```python
from build123d import *

# Parameters (mm, degrees)
SKETCH1_W               = 390
SKETCH1_H               = 120
SKETCH1_R               = 3.2
BOSS_EXTRUDE1_DEPTH     = 2.03
EDGE_FLANGE1_DEPTH      = 120
EDGE_FLANGE1_BEND_DEPTH = 120
CUT_EXTRUDE1_REACH      = 210.681
CUT_EXTRUDE2_DEPTH      = 209.447861347
CUT_EXTRUDE2_DEPTH_BACK = 209.447861347
SKETCH19_R              = 2.5
SKETCH20_R              = 3.35
CUT_EXTRUDE3_DEPTH      = 209.447861347
SKETCH21_R              = 3.175
CUT_EXTRUDE4_DEPTH      = 209.681312053


# Sheet-metal steps are written as plain solids
with BuildPart() as part:
    # Sketch1 → Boss-Extrude1 (new body)
    with BuildSketch(Plane(origin=(0, 0, 0), x_dir=(1, 0, 0), z_dir=(0, 1, 0))):
        Rectangle(SKETCH1_W, SKETCH1_H)
        with Locations(Location((0, 50, 0), (0, 0, 270))):
            Circle(SKETCH1_R, mode=Mode.SUBTRACT)
        with Locations(Location((-185, 50, 0), (0, 0, 270))):
            Circle(SKETCH1_R, mode=Mode.SUBTRACT)
        with Locations(Location((-185, -50, 0), (0, 0, 270))):
            Circle(SKETCH1_R, mode=Mode.SUBTRACT)
        with Locations(Location((0, -50, 0), (0, 0, 270))):
            Circle(SKETCH1_R, mode=Mode.SUBTRACT)
        with Locations(Location((185, -50, 0), (0, 0, 270))):
            Circle(SKETCH1_R, mode=Mode.SUBTRACT)
        with Locations(Location((185, 50, 0), (0, 0, 270))):
            Circle(SKETCH1_R, mode=Mode.SUBTRACT)
    extrude(amount=-BOSS_EXTRUDE1_DEPTH)

    # Edge-Flange1 section (across the edge) → Edge-Flange1 (add)
    with BuildSketch(Plane(origin=(-196.27, 0, -60), x_dir=(1, 0, 0), z_dir=(0, 0, 1))):
        with BuildLine():
            Line((-2.03, 1.27), (-2.03, 22.97))
            Line((-2.03, 22.97), (0, 22.97))
            Line((0, 22.97), (0, 1.27))
            ThreePointArc((0, 1.27), (0.371974388, 0.371974388), (1.27, 0))
            Line((1.27, 0), (1.27, -2.03))
            ThreePointArc((1.27, -2.03), (-1.063452378, -1.063452378), (-2.03, 1.27))
        make_face()
    extrude(amount=EDGE_FLANGE1_DEPTH)

    # Edge-Flange1 section 2 (across the edge) → Edge-Flange1 bend (add)
    with BuildSketch(Plane(origin=(196.27, 0, 60), x_dir=(-1, 0, 0), z_dir=(0, 0, -1))):
        with BuildLine():
            Line((-2.03, 1.27), (-2.03, 22.97))
            Line((-2.03, 22.97), (0, 22.97))
            Line((0, 22.97), (0, 1.27))
            ThreePointArc((0, 1.27), (0.371974388, 0.371974388), (1.27, 0))
            Line((1.27, 0), (1.27, -2.03))
            ThreePointArc((1.27, -2.03), (-1.063452378, -1.063452378), (-2.03, 1.27))
        make_face()
    extrude(amount=EDGE_FLANGE1_BEND_DEPTH)

    # Sketch18 → Cut-Extrude1 (cut, up to next)
    with BuildSketch(Plane.XZ.offset(2.03), mode=Mode.PRIVATE) as cut_extrude1_sk1:
        with BuildLine():
            Line((-157.5, -37.5), (-27.5, -37.5))
            ThreePointArc((-27.5, -37.5), (-23.964466094, -36.035533906), (-22.5, -32.5))
            Line((-22.5, -32.5), (-22.5, 32.5))
            ThreePointArc((-22.5, 32.5), (-23.964466094, 36.035533906), (-27.5, 37.5))
            Line((-27.5, 37.5), (-157.5, 37.5))
            ThreePointArc((-157.5, 37.5), (-161.035533906, 36.035533906), (-162.5, 32.5))
            Line((-162.5, 32.5), (-162.5, -32.5))
            ThreePointArc((-162.5, -32.5), (-161.035533906, -36.035533906), (-157.5, -37.5))
        make_face()
    cut_extrude1_tool1 = extrude(cut_extrude1_sk1.sketch, amount=-CUT_EXTRUDE1_REACH, mode=Mode.PRIVATE) & part.part
    # Sketch18 → Cut-Extrude1 (cut, up to next)
    with BuildSketch(Plane.XZ.offset(2.03), mode=Mode.PRIVATE) as cut_extrude1_sk2:
        with BuildLine():
            Line((22.5, -32.5), (22.5, 32.5))
            ThreePointArc((22.5, 32.5), (23.964466094, 36.035533906), (27.5, 37.5))
            Line((27.5, 37.5), (157.5, 37.5))
            ThreePointArc((157.5, 37.5), (161.035533906, 36.035533906), (162.5, 32.5))
            Line((162.5, 32.5), (162.5, -32.5))
            ThreePointArc((162.5, -32.5), (161.035533906, -36.035533906), (157.5, -37.5))
            Line((157.5, -37.5), (27.5, -37.5))
            ThreePointArc((27.5, -37.5), (23.964466094, -36.035533906), (22.5, -32.5))
        make_face()
    cut_extrude1_tool2 = extrude(cut_extrude1_sk2.sketch, amount=-CUT_EXTRUDE1_REACH, mode=Mode.PRIVATE) & part.part
    add(cut_extrude1_tool1.solids().sort_by_distance((-92.5, -2.03, 0))[0], mode=Mode.SUBTRACT)
    add(cut_extrude1_tool2.solids().sort_by_distance((92.5, -2.03, 0))[0], mode=Mode.SUBTRACT)

    # Sketch19 → Cut-Extrude2 (cut, two sides: drawn at the far end of the back side and taken through both)
    with BuildSketch(Plane(origin=(0, 0, 0), x_dir=(0, 0, -1), z_dir=(1, 0, 0)).offset(-CUT_EXTRUDE2_DEPTH_BACK)):
        with Locations((-47.5, 15.65)):
            Circle(SKETCH19_R)
        with Locations((0, 15.65)):
            Circle(SKETCH19_R)
        with Locations((47.5, 15.65)):
            Circle(SKETCH19_R)
    extrude(amount=CUT_EXTRUDE2_DEPTH + CUT_EXTRUDE2_DEPTH_BACK, mode=Mode.SUBTRACT)

    # Sketch20 → Cut-Extrude3 (cut, through all)
    with BuildSketch(Plane(origin=(0, 0, 0), x_dir=(1, 0, 0), z_dir=(0, 1, 0))):
        with Locations(Location((-92.5, -48.75, 0), (0, 0, 270))):
            Circle(SKETCH20_R)
        with Locations(Location((92.5, -48.75, 0), (0, 0, 90))):
            Circle(SKETCH20_R)
        with Locations(Location((92.5, 48.75, 0), (0, 0, 270))):
            Circle(SKETCH20_R)
        with Locations(Location((-92.5, 48.75, 0), (0, 0, 90))):
            Circle(SKETCH20_R)
    extrude(amount=-CUT_EXTRUDE3_DEPTH, mode=Mode.SUBTRACT)

    # Sketch21 → Cut-Extrude4 (cut, through all)
    with BuildSketch(Plane.XZ.offset(2.03)):
        with Locations(Location((-180, 0, 0), (0, 0, 270))):
            Circle(SKETCH21_R)
    extrude(amount=-CUT_EXTRUDE4_DEPTH, mode=Mode.SUBTRACT)


solid = part.part
```
Work out the finished part from the listing and answer in its coordinate system (mm). A direction names the side the tool comes from. Give positions to 0.01 mm unless a question says otherwise; leave off trailing zeros. Order: outer loops, then holes, each group sorted by start corner. A loop starts at its lowest first (then second) coordinate and runs counter-clockwise, first axis right, second up. Notation, with made-up numbers: (-29.5, 77) - (-24.5, 77) arc R25 cw to (-24.5, 114) - close; hole circle Ø2 at (-6.75, -16). An arc over 180 degrees is marked (long way). One line per item, written item: value. Start each with the question number.
1. Section B-B, the plane x = 92.5 is taken. Write down the section's boundary in (y, z), then the cut area to 3 significant figures.
2. Each of these flat-tipped pins is pushed along its axis until it touches: pin 1 Ø10 at (x, z) = (-180, 0) entering from +Y; pin 2 Ø0.6 at (y, z) = (-0.5, -11) entering from +X; pin 3 Ø1.6 at (y, z) = (-1, -3) entering from -X. Where does it stop, or does it pass through?
3. Section A-A, the plane x = -153 is taken. Write down the section's boundary in (y, z).
4. Consider line 1 (Z direction, x = -197.2, y = 15.65); line 2 (X direction, y = 1.5, z = -9); line 3 (Z direction, x = 185, y = -0.65). Determine where each line is inside the solid, lowest interval first.
5. Which of the six approach directions +Z, -Z, +X, -X, +Y, -Y give full straight-line access (tool end or side, diameter ignored) to faces 5 (the face through (196.27, 12, 1)), 6 (the face through (-3, -2.03, -1))?
6. Section C-C, the plane y = 6.75 is taken. Write down the section's boundary in (x, z).
7. For a pull along Z with two mould halves and no side action, classify faces 1 (the face through (188.173, -1.001, 49.583)), 2 (the face through (-1, -1, 60)), 3 (the face through (-176.85, -1.03, 0.41)), 4 (the face through (-3, 0, -1)) as released by +Z, released by -Z, zero draft, split by the parting line, or undercut.
Filled sheet:
1. outline: (-2.03, -60) - (0, -60) - (0, -52.1) - (-2.03, -52.1) - close; (-2.03, -45.4) - (0, -45.4) - (0, -37.5) - (-2.03, -37.5) - close; (-2.03, 37.5) - (0, 37.5) - (0, 45.4) - (-2.03, 45.4) - close; (-2.03, 52.1) - (0, 52.1) - (0, 60) - (-2.03, 60) - close
1. area: 64.1 mm²
2. pin 1: y = 0
2. pin 2: x = 197.95
2. pin 3: x = -197.95
3. outline: (-2.03, -60) - (0, -60) - (0, -37.5) - (-2.03, -37.5) - close; (-2.03, 37.5) - (0, 37.5) - (0, 60) - (-2.03, 60) - close
4. line 1: -60 to -50, -45 to -2.5, 2.5 to 45, 50 to 60
4. line 2: -198.3 to -196.27, 196.27 to 198.3
4. line 3: -60 to -53.2, -46.8 to 46.8, 53.2 to 60
5. face 5: +Z, -Z, +Y
5. face 6: +Z, -Z, +X, -X, -Y
6. outline: (-198.3, -60) - (-196.27, -60) - (-196.27, 60) - (-198.3, 60) - close; (196.27, -60) - (198.3, -60) - (198.3, 60) - (196.27, 60) - close
7. face 1: undercut
7. face 2: released by +Z
7. face 3: undercut
7. face 4: zero draft
